Work out the finished part from the listing and answer in its coordinate system (mm). Give positions to 0.01 mm unless a question says otherwise; leave off trailing zeros. Loops run counter-clockwise (first coordinate to the right, second up) from the corner with the lowest first, then second, coordinate; pieces in that order, holes last.
from build123d import *

# Parameters (mm, degrees)
F0_R     = 10.5918
F0_R_2   = 11.0617
F1_DEPTH = 2.54


with BuildPart() as f1:
    # F0 (on Top) → F1 (new body)
    with BuildSketch(Plane.XY):
        Polygon((37.805012, 12.867026), (0, 12.867026), (-38.394988, 12.867026), (-38.394988, -15.072974), (37.805012, -15.072974), align=None)
        with Locations((-25.4, 0)):
            Circle(F0_R, mode=Mode.SUBTRACT)
        with BuildLine():
            ThreePointArc((0, 10.6045), (7.498514, 7.498514), (10.6045, 0))
            ThreePointArc((10.6045, 0), (0, -10.6045), (-10.6045, 0))
            ThreePointArc((-10.6045, 0), (-7.498514, 7.498514), (0, 10.6045))
        make_face(mode=Mode.SUBTRACT)
        with BuildLine():
            ThreePointArc((36.0172, 0), (25.4, -10.6172), (14.7828, 0))
            ThreePointArc((14.7828, 0), (25.4, 10.6172), (36.0172, 0))
        make_face(mode=Mode.SUBTRACT)
        Polygon((-38.394988, 12.867026), (0, 12.867026), (37.805012, 12.867026), (37.805012, 38.267026), (-38.394988, 38.267026), align=None)
        with Locations((-25.4, 25.4)):
            Circle(F0_R_2, mode=Mode.SUBTRACT)
        with BuildLine():
            ThreePointArc((11.049, 25.4), (7.812823, 17.587177), (0, 14.351))
            ThreePointArc((0, 14.351), (-7.812823, 17.587177), (-11.049, 25.4))
            ThreePointArc((-11.049, 25.4), (0, 36.449), (11.049, 25.4))
        make_face(mode=Mode.SUBTRACT)
        with BuildLine():
            ThreePointArc((36.4363, 25.4), (25.4, 14.3637), (14.3637, 25.4))
            ThreePointArc((14.3637, 25.4), (25.4, 36.4363), (36.4363, 25.4))
        make_face(mode=Mode.SUBTRACT)
    extrude(amount=F1_DEPTH)


solid = f1.part
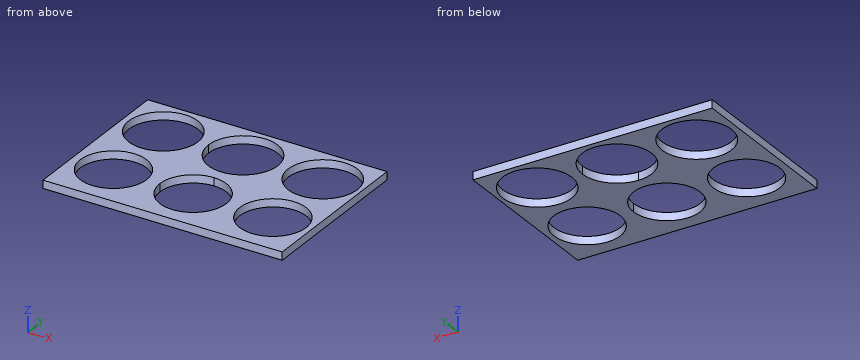
Item 1: Find section C-C, the plane y = 31. Write down the section's boundary in (x, z), plus the area to 3 significant figures.
Item 2: Find section D-D, the plane y = 3.5. Write down the section's boundary in (x, z), plus the area to 3 significant figures.
Item 3: Find section B-B, the plane z = 1.15. Write down the section's boundary in (x, y).
Item 4: Flat-ended cylindrical pins translate along their axes: pin 1 Ø5 at (x, y) = (-5.5, 22) entering from +Z; pin 2 Ø3 at (x, y) = (-12, -7.5) entering from -Z. Find the tip coordinate at first contact, or state that the pin passes through.
Item 5: Find section A-A, the plane x = -25.4. Write down the section's boundary in (y, z), plus the area to 3 significant figures.
Item 6: Consider line 1 (X direction, y = 25, z = 1.8); line 2 (Y direction, x = -25.4, z = 1.75); line 3 (Y direction, x = 25.4, z = 0.8). Determine where each line is inside the solid, lowest interval first.
Ans:
1. outline: (-38.39, 0) - (-34.94, 0) - (-34.94, 2.54) - (-38.39, 2.54) - close; (-15.86, 0) - (-9.52, 0) - (-9.52, 2.54) - (-15.86, 2.54) - close; (9.52, 0) - (15.89, 0) - (15.89, 2.54) - (9.52, 2.54) - close; (34.91, 0) - (37.81, 0) - (37.81, 2.54) - (34.91, 2.54) - close
1. area: 48.4 mm2
2. outline: (-38.39, 0) - (-35.4, 0) - (-35.4, 2.54) - (-38.39, 2.54) - close; (-15.4, 0) - (-10.01, 0) - (-10.01, 2.54) - (-15.4, 2.54) - close; (10.01, 0) - (15.38, 0) - (15.38, 2.54) - (10.01, 2.54) - close; (35.42, 0) - (37.81, 0) - (37.81, 2.54) - (35.42, 2.54) - close
2. area: 41.0 mm2
3. outline: (-38.39, -15.07) - (37.81, -15.07) - (37.81, 38.27) - (-38.39, 38.27) - close; hole circle Ø22.12 at (-25.4, 25.4); hole circle Ø21.18 at (-25.4, 0); hole circle Ø21.21 at (0, 0); hole (0, 14.35) arc R11.05 ccw to (11.05, 25.4) arc R11.05 ccw (long way) to start; hole circle Ø22.07 at (25.4, 25.4); hole circle Ø21.23 at (25.4, 0)
4. pin 1: passes through
4. pin 2: stops at z = 0
5. outline: (-15.07, 0) - (-10.59, 0) - (-10.59, 2.54) - (-15.07, 2.54) - close; (10.59, 0) - (14.34, 0) - (14.34, 2.54) - (10.59, 2.54) - close; (36.46, 0) - (38.27, 0) - (38.27, 2.54) - (36.46, 2.54) - close
5. area: 25.5 mm2
6. line 1: x = -38.39 to -36.45, -14.35 to -11.04, 11.04 to 14.37, 36.43 to 37.81
6. line 2: y = -15.07 to -10.59, 10.59 to 14.34, 36.46 to 38.27
6. line 3: y = -15.07 to -10.62, 10.62 to 14.36, 36.44 to 38.27
